The figure shows three views and two pictorial views of one solid part (mm, origin at its lowest corner). Answer the questions. A direction names the side the tool comes from. Give positions to 0.01 mm unless a question says otherwise; leave off trailing zeros. Write each loop counter-clockwise with the first axis right and the second up, starting at its lowest first coordinate (ties: lowest second). Pieces come first, ordered by that corner, then holes. Notation, with made-up numbers: (41.25, 67) - (72.25, 67) arc R25 cw to (72.25, 102) - close; hole circle Ø9 at (48.5, -24). An arc over 180 degrees is marked (long way). One line per question, with ' | ' between items. Start each with the question number.
1. A cutting plane is placed at B-B (z = 7.5). Determine the outline of the cut face in (x, y), then the cut area to 3 significant figures.
2. For the marked faces 1 and 2, determine the directions among +Z, -Z, +X, -X, +Y, -Y from which every point of the face is accessible in a straight line to the end or side of a thin tool.
3. A cutting plane is placed at A-A (x = 5). Determine the outline of the cut face in (y, z), then the cut area to 3 significant figures.
4. A cutting plane is placed at C-C (y = 6.5). Determine the outline of the cut face in (x, z).
5. The mould has two halves that part along Z. Classify the marked faces 3, 4 and 5: +Z half, -Z half, draft (parallel to the pull), parting line (faces both ways), or undercut.
6. A cutting plane is placed at D-D (x = 9). Determine the outline of the cut face in (y, z).
7. Given P1, Ø2, axis at y = 11.5, z = 8, coming from the +X side; P2, Ø2, axis at x = 8.5, y = 13, coming from the +Z side, each flat-ended and moving along its own axis, determine where each tip first touches the part or whether it passes through.
8. Find the intervals of material crossed by L1, parallel to Z at x = 5, y = 7.5; L2, parallel to X at y = 4.5, z = 7.5; L3, parallel to Y at x = 8.75, z = 2, in increasing order. Write a range as from..to.
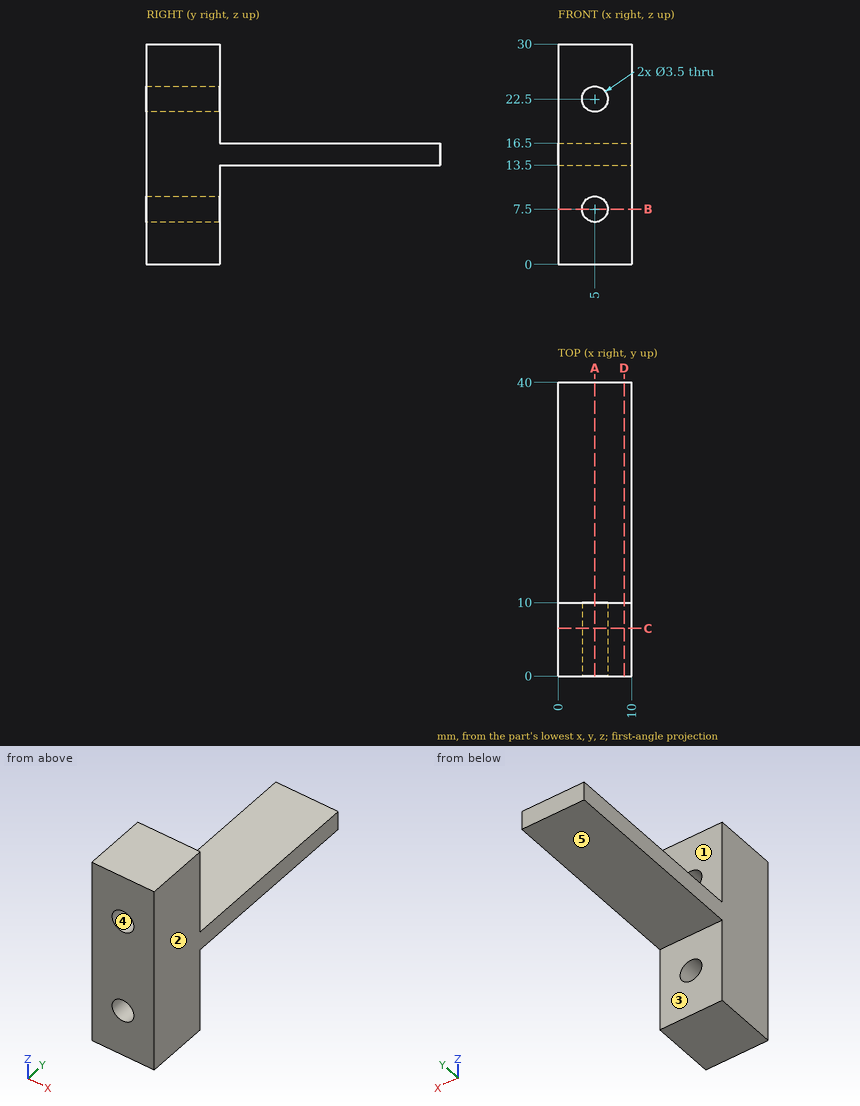
Determined:
1) outline: (0, 0) - (3.25, 0) - (3.25, 10) - (0, 10) - close; (6.75, 0) - (10, 0) - (10, 10) - (6.75, 10) - close | area: 65.0 mm2
2) face 1: +Z, +X, -X, +Y | face 2: +Z, -Z, +X, +Y, -Y
3) outline: (0, 0) - (10, 0) - (10, 5.75) - (0, 5.75) - close; (0, 9.25) - (10, 9.25) - (10, 13.5) - (40, 13.5) - (40, 16.5) - (10, 16.5) - (10, 20.75) - (0, 20.75) - close; (0, 24.25) - (10, 24.25) - (10, 30) - (0, 30) - close | area: 320 mm2
4) outline: (0, 0) - (10, 0) - (10, 30) - (0, 30) - close; hole circle Ø3.5 at (5, 7.5); hole circle Ø3.5 at (5, 22.5)
5) face 3: draft | face 4: undercut | face 5: -Z half
6) outline: (0, 0) - (10, 0) - (10, 13.5) - (40, 13.5) - (40, 16.5) - (10, 16.5) - (10, 30) - (0, 30) - close
7) P1: through | P2: z = 16.5
8) L1: 0..5.75, 9.25..20.75, 24.25..30 | L2: 0..3.25, 6.75..10 | L3: 0..10
